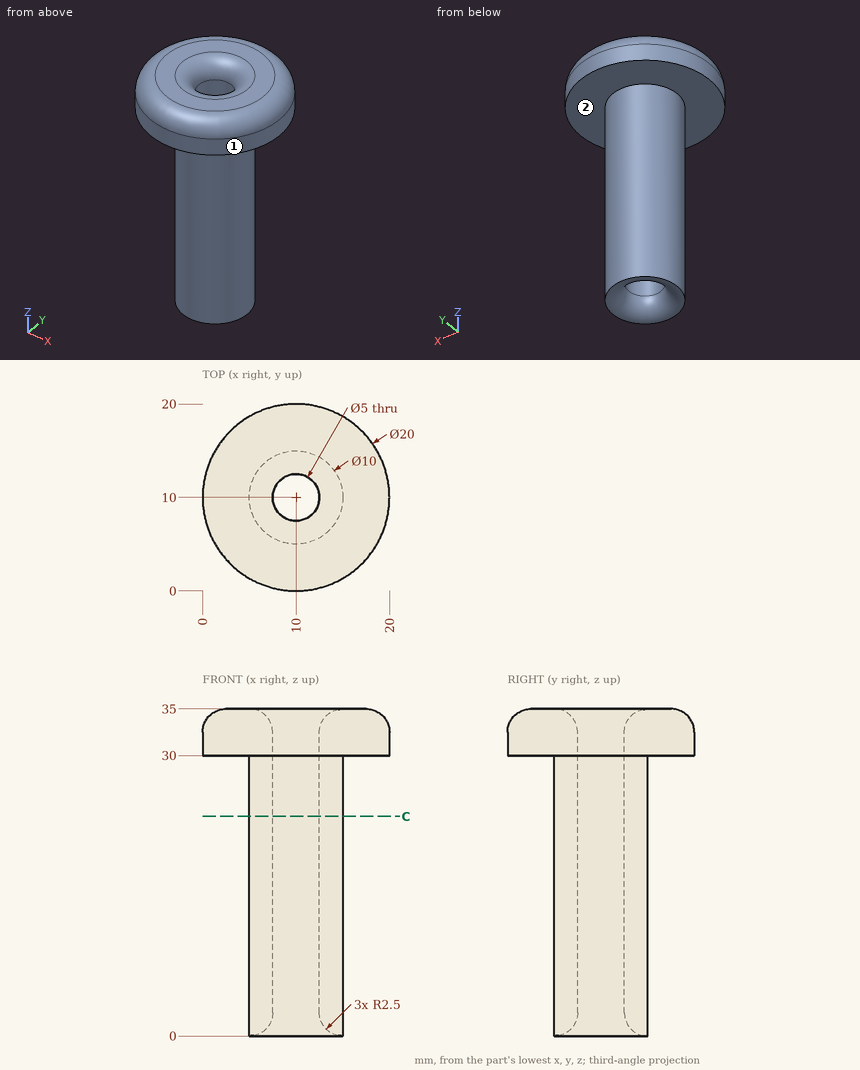
Here's the drawing with two shaded views (mm, measured from the low corner). I have some questions. A direction names the side the tool comes from. Round coordinates to 2 decimals unless told otherwise and drop trailing zeros. Loops run counter-clockwise (first coordinate to the right, second up) from the corner with the lowest first, then second, coordinate; pieces in that order, holes last. Notation, with made-up numbers: (-12, 7) -> (0, 7) arc R15 ccw to (0, 13) -> close; hole circle Ø11 at (76.25, -15). An arc over 180 degrees is marked (long way). Answer as CSV lines item,"result". Start each with the question number.
1. Imagine slicing it at C-C on z = 23.5. Write out the boundary of the cut face in (x, y).
2. I need wall thicknesses on probe 1 along Y at (x, z) = (10, 12); probe 2 along X at (y, z) = (10.5, 19.5). Which ranges of each line are inside material? Lowest first, please. Write a range as from..to.
3. I'm going to push flat-ended pins straight in: P1, Ø8, axis at x = 15, z = 16, coming from the +Y side; P2, Ø5, axis at y = 7.5, z = 8, coming from the -X side; P3, Ø6, axis at x = 6.5, z = 22.5, coming from the -Y side. Where does each tip first touch, or does it pass through?
4. For the marked faces 1 and 2, which set-ups out of +Z, -Z, +X, -X, +Y, -Y let a thin tool reach every point of the face, with its end or its side?
Solution:
1,outline,"circle Ø10 at (10, 10); hole circle Ø5 at (10, 10)"
2,probe 1,"5..7.5, 12.5..15"
2,probe 2,"5.03..7.55, 12.45..14.97"
3,P1,"y = 14.9"
3,P2,"x = 5"
3,P3,"y = 5.03"
4,face 1,"+Z, -Z"
4,face 2,"-Z"
